Here's how the part is built. I have some questions about the finished solid (model axes, mm). Face numbers are marked on the shaded views. A direction names the side the tool comes from. Round coordinates to 2 decimals unless told otherwise and drop trailing zeros. Loops run counter-clockwise (first coordinate to the right, second up) from the corner with the lowest first, then second, coordinate; pieces in that order, holes last. Notation, with made-up numbers: M -19,12.5 L 17,12.5 A26 ccw 17,32.5 Z; hole C 18.5,57 d6. An arc over 180 degrees is marked long. Write each question's results on one line, items separated by ' | '. Start each with the question number.
```python
from build123d import *

# Parameters (mm, degrees)
PAD_DEPTH    = 1
SKETCH001_W  = 20
SKETCH001_H  = 16
PAD001_DEPTH = 1.6
PAD002_DEPTH = 2
FILLET_R     = 2
CHAMFER_SIZE = 2.4
FILLET001_R  = 1.2
FILLET002_R  = 2
FILLET003_R  = 2


with BuildPart() as part:
    # Sketch → Pad (new body)
    with BuildSketch(Plane.XY):
        Polygon((-10, 8), (-10, -8), (-5, -8), (-5, -26.5), (5, -26.5), (5, -8), (10, -8), (10, 8), (5, 8), (5, 26.5), (-5, 26.5), (-5, 8), align=None)
    extrude(amount=PAD_DEPTH)

    # Sketch001 (on Face14 of Pad) → Pad001 (join)
    with BuildSketch(Plane.XY.offset(1)):
        Rectangle(SKETCH001_W, SKETCH001_H)
    extrude(amount=PAD001_DEPTH)

    # Sketch002 (on Face8 of Pad001) → Pad002 (join)
    with BuildSketch(Plane.XY.offset(1)):
        Polygon((-5, 26.5), (5, 26.5), (5, 22.5), (0, 19.5), (-5, 22.5), align=None)
    pad002 = extrude(amount=PAD002_DEPTH)

    # Mirrored: Pad002 across Sketch002 H_Axis
    add(pad002.mirror(Plane(origin=(0, 0, 1), x_dir=(0, 0, 1), z_dir=(0, 1, 0))))

    # Fillet
    fillet_edges = [part.edges().sort_by_distance(p)[0] for p in [
        (5, -8, 0.5),
        (-5, -8, 0.5),
        (-5, 8, 0.5),
        (5, 8, 0.5),
    ]]
    fillet(fillet_edges, radius=FILLET_R)

    # Chamfer
    chamfer_edges = [part.edges().sort_by_distance(p)[0] for p in [
        (0, 26.5, 3),
        (0, -26.5, 3),
    ]]
    chamfer(chamfer_edges, length=CHAMFER_SIZE)

    # Fillet001
    fillet001_edges = [part.edges().sort_by_distance(p)[0] for p in [
        (0, 8, 1),
        (0, -8, 1),
    ]]
    fillet(fillet001_edges, radius=FILLET001_R)

    # Fillet002
    fillet002_edges = [part.edges().sort_by_distance(p)[0] for p in [
        (10, 0, 0),
        (-10, 0, 0),
    ]]
    fillet(fillet002_edges, radius=FILLET002_R)

    # Fillet003
    fillet003_edges = [part.edges().sort_by_distance(p)[0] for p in [
        (-5, -26.5, 0.3),
        (5, -26.5, 0.3),
        (-5, 26.5, 0.3),
        (5, 26.5, 0.3),
    ]]
    fillet(fillet003_edges, radius=FILLET003_R)


solid = part.part
```
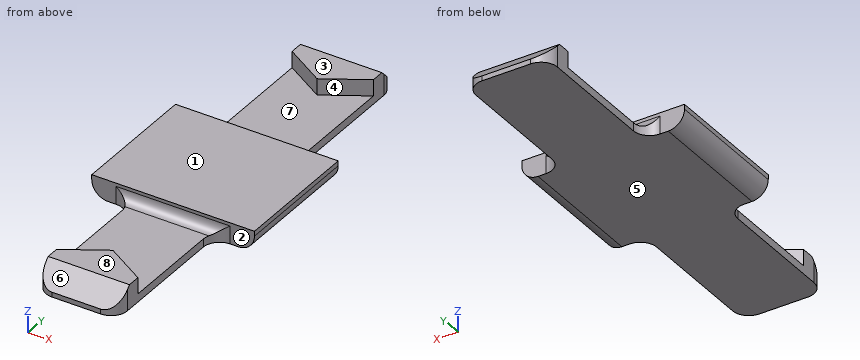
Item 1: If we section it at A-A on y = -3: Please give me the cut outline in (x, z), and give its area (3 significant figures).
Item 2: Which directions (+Z, -Z, +X, -X, +Y, -Y) give clear straight access to the entire face, cutting with the end or side of a thin tool? Please do the marked faces 1, 2, 3, 4 and 5.
Item 3: If we section it at B-B on y = 16: Please give me the cut outline in (x, z).
Item 4: If we mould it in two halves opening along Y, with no side actions, what happens to the marked faces 6, 7 and 8? For each: released by +Y, released by -Y, zero draft, split by the parting line, or undercut.
Item 5: I'm going to push flat-ended pins straight in: pin 1 (0.8 mm diameter, centred on x = -3.5, z = 0.5, fed in from +Y); pin 2 (0.9 mm diameter, centred on y = -16, z = 2, fed in from -X); pin 3 (8.5 mm diameter, centred on x = -0.5, y = 13.5, fed in from +Z); pin 4 (1.5 mm diameter, centred on y = 19, z = 1, fed in from -X). Where does each tip first touch, or does it pass through?
Item 6: I need wall thicknesses on L1, parallel to Y at x = 1, z = 1.85; L2, parallel to Y at x = -3.5, z = 2.4; L3, parallel to Z at x = 2, y = 15. Which ranges of each line are inside material? Lowest first, please.
Numbers:
1) outline: M -10,2 A2 ccw -8,0 L 8,0 A2 ccw 10,2 L 10,2.6 L -10,2.6 Z | area: 50.3 mm²
2) face 1: +Z, +X, -X | face 2: +Z | face 3: +Z, +X, -X, +Y, -Y | face 4: +Z, +X | face 5: -Z, +X, -X, +Y, -Y
3) outline: M -5,0 L 5,0 L 5,1 L -5,1 Z
4) face 6: released by -Y | face 7: undercut | face 8: zero draft
5) pin 1: y = 26.5 | pin 2: through | pin 3: z = 1 | pin 4: x = -5
6) L1: -25.25 to -20.1, -8.05 to 8.05, 20.1 to 25.25 | L2: -24.7 to -21.6, -8 to 8, 21.6 to 24.7 | L3: 0 to 1
